from build123d import *

# Parameters (mm, degrees)
F0_R     = 11.35
F1_DEPTH = 2
F2_R     = 2.6
F3_DEPTH = 25


# Not quite as in the source:
# - a feature names something its author has since deleted; it is built from what else it names


with BuildPart() as f1:
    # F0 (on Top) → F1 (new body)
    with BuildSketch(Plane.XY):
        Circle(F0_R)
    extrude(amount=F1_DEPTH)

    # F2 (on face) → F3 (cut)
    with BuildSketch(Plane.XY.offset(2)):
        with BuildLine():
            ThreePointArc((9.1045560576, 6.7771350137), (7.7736409673, 8.2700064155), (6.2013506213, 9.506090178))
            ThreePointArc((6.2013506213, 9.506090178), (6.4038363916, 6.8127365625), (9.1045560576, 6.7771350137))
        make_face()
        with BuildLine():
            ThreePointArc((9.1045560576, 6.7771350137), (9.5987204424, 7.4520303097), (9.7736409673, 8.2700064155))
            ThreePointArc((9.7736409673, 8.2700064155), (8.4276361156, 10.1600567709), (6.2013506213, 9.506090178))
            ThreePointArc((6.2013506213, 9.506090178), (7.7736409673, 8.2700064155), (9.1045560576, 6.7771350137))
        make_face()
        with BuildLine():
            ThreePointArc((0.6174820868, 11.3331908954), (2.1395167155, 9.1019211282), (4.4962093293, 10.4214491155))
            ThreePointArc((4.4962093293, 10.4214491155), (2.5971673498, 11.0488561289), (0.6174820868, 11.3331908954))
        make_face()
        with BuildLine():
            ThreePointArc((0.6174820868, 11.3331908954), (2.5971673498, 11.0488561289), (4.4962093293, 10.4214491155))
            ThreePointArc((4.4962093293, 10.4214491155), (4.5717665445, 10.73111721), (4.5971673498, 11.0488561289))
            ThreePointArc((4.5971673498, 11.0488561289), (2.7396971257, 13.04377098), (0.6174820868, 11.3331908954))
        make_face()
        with BuildLine():
            ThreePointArc((-5.1318402741, 10.1235722648), (-3.2752151616, 10.8671737653), (-1.3168930579, 11.2733443429))
            ThreePointArc((-1.3168930579, 11.2733443429), (-3.8523455866, 12.7820942526), (-5.1318402741, 10.1235722648))
        make_face()
        with BuildLine():
            ThreePointArc((-1.2752151616, 10.8671737653), (-1.2856619194, 11.0713254155), (-1.3168930579, 11.2733443429))
            ThreePointArc((-1.3168930579, 11.2733443429), (-3.2752151616, 10.8671737653), (-5.1318402741, 10.1235722648))
            ThreePointArc((-5.1318402741, 10.1235722648), (-2.8965663963, 8.9033445689), (-1.2752151616, 10.8671737653))
        make_face()
        with BuildLine():
            ThreePointArc((-9.506090178, 6.2013506213), (-8.2700064155, 7.7736409673), (-6.7771350137, 9.1045560576))
            ThreePointArc((-6.7771350137, 9.1045560576), (-9.7272762684, 9.143445543), (-9.506090178, 6.2013506213))
        make_face()
        with BuildLine():
            ThreePointArc((-6.2700064155, 7.7736409673), (-6.4010838912, 8.4857705891), (-6.7771350137, 9.1045560576))
            ThreePointArc((-6.7771350137, 9.1045560576), (-8.2700064155, 7.7736409673), (-9.506090178, 6.2013506213))
            ThreePointArc((-9.506090178, 6.2013506213), (-7.3959833966, 5.97472914), (-6.2700064155, 7.7736409673))
        make_face()
        with BuildLine():
            ThreePointArc((-11.3331908954, 0.6174820868), (-11.0488561289, 2.5971673498), (-10.4214491155, 4.4962093293))
            ThreePointArc((-10.4214491155, 4.4962093293), (-12.9957911296, 3.0548179842), (-11.3331908954, 0.6174820868))
        make_face()
        with BuildLine():
            ThreePointArc((-9.0488561289, 2.5971673498), (-9.427928304, 3.7687444863), (-10.4214491155, 4.4962093293))
            ThreePointArc((-10.4214491155, 4.4962093293), (-11.0488561289, 2.5971673498), (-11.3331908954, 0.6174820868))
            ThreePointArc((-11.3331908954, 0.6174820868), (-9.7390220808, 1.0857657597), (-9.0488561289, 2.5971673498))
        make_face()
        with BuildLine():
            ThreePointArc((11.2733443429, 1.3168930579), (10.8671737653, 3.2752151616), (10.1235722648, 5.1318402741))
            ThreePointArc((10.1235722648, 5.1318402741), (8.952253278, 2.6980847366), (11.2733443429, 1.3168930579))
        make_face()
        with BuildLine():
            ThreePointArc((12.8671737653, 3.2752151616), (11.9880655975, 4.9315972131), (10.1235722648, 5.1318402741))
            ThreePointArc((10.1235722648, 5.1318402741), (10.8671737653, 3.2752151616), (11.2733443429, 1.3168930579))
            ThreePointArc((11.2733443429, 1.3168930579), (12.4183573707, 2.0127455887), (12.8671737653, 3.2752151616))
        make_face()
        with BuildLine():
            ThreePointArc((10.4214491155, -4.4962093293), (11.0488561289, -2.5971673498), (11.3331908954, -0.6174820868))
            ThreePointArc((11.3331908954, -0.6174820868), (9.1019211282, -2.1395167155), (10.4214491155, -4.4962093293))
        make_face()
        with BuildLine():
            ThreePointArc((13.0488561289, -2.5971673498), (12.560257719, -1.2873333018), (11.3331908954, -0.6174820868))
            ThreePointArc((11.3331908954, -0.6174820868), (11.0488561289, -2.5971673498), (10.4214491155, -4.4962093293))
            ThreePointArc((10.4214491155, -4.4962093293), (12.2204332653, -4.2180951747), (13.0488561289, -2.5971673498))
        make_face()
        with BuildLine():
            ThreePointArc((-4.4962093293, -10.4214491155), (-3.0548179842, -12.9957911296), (-0.6174820868, -11.3331908954))
            ThreePointArc((-0.6174820868, -11.3331908954), (-2.5971673498, -11.0488561289), (-4.4962093293, -10.4214491155))
        make_face()
        with BuildLine():
            ThreePointArc((-4.4962093293, -10.4214491155), (-2.5971673498, -11.0488561289), (-0.6174820868, -11.3331908954))
            ThreePointArc((-0.6174820868, -11.3331908954), (-0.6022524988, -11.1913859047), (-0.5971673498, -11.0488561289))
            ThreePointArc((-0.5971673498, -11.0488561289), (-2.2794284309, -9.0742569343), (-4.4962093293, -10.4214491155))
        make_face()
        with BuildLine():
            ThreePointArc((-10.1235722648, -5.1318402741), (-10.8671737653, -3.2752151616), (-11.2733443429, -1.3168930579))
            ThreePointArc((-11.2733443429, -1.3168930579), (-12.7820942526, -3.8523455866), (-10.1235722648, -5.1318402741))
        make_face()
        with BuildLine():
            ThreePointArc((-8.8671737653, -3.2752151616), (-9.6047041924, -1.7240315562), (-11.2733443429, -1.3168930579))
            ThreePointArc((-11.2733443429, -1.3168930579), (-10.8671737653, -3.2752151616), (-10.1235722648, -5.1318402741))
            ThreePointArc((-10.1235722648, -5.1318402741), (-9.2107917138, -4.3961069938), (-8.8671737653, -3.2752151616))
        make_face()
        with BuildLine():
            ThreePointArc((-6.2013506213, -9.506090178), (-7.7736409673, -8.2700064155), (-9.1045560576, -6.7771350137))
            ThreePointArc((-9.1045560576, -6.7771350137), (-9.143445543, -9.7272762684), (-6.2013506213, -9.506090178))
        make_face()
        with BuildLine():
            ThreePointArc((-5.7736409673, -8.2700064155), (-6.9556648615, -6.4449269404), (-9.1045560576, -6.7771350137))
            ThreePointArc((-9.1045560576, -6.7771350137), (-7.7736409673, -8.2700064155), (-6.2013506213, -9.506090178))
            ThreePointArc((-6.2013506213, -9.506090178), (-5.8835906119, -8.9240015638), (-5.7736409673, -8.2700064155))
        make_face()
        with BuildLine():
            ThreePointArc((6.7771350137, -9.1045560576), (8.2700064155, -7.7736409673), (9.506090178, -6.2013506213))
            ThreePointArc((9.506090178, -6.2013506213), (6.8127365625, -6.4038363916), (6.7771350137, -9.1045560576))
        make_face()
        with BuildLine():
            ThreePointArc((10.2700064155, -7.7736409673), (10.0689182428, -6.8996179484), (9.506090178, -6.2013506213))
            ThreePointArc((9.506090178, -6.2013506213), (8.2700064155, -7.7736409673), (6.7771350137, -9.1045560576))
            ThreePointArc((6.7771350137, -9.1045560576), (8.9821360372, -9.6425634916), (10.2700064155, -7.7736409673))
        make_face()
        with BuildLine():
            ThreePointArc((1.3168930579, -11.2733443429), (3.2752151616, -10.8671737653), (5.1318402741, -10.1235722648))
            ThreePointArc((5.1318402741, -10.1235722648), (2.6980847366, -8.952253278), (1.3168930579, -11.2733443429))
        make_face()
        with BuildLine():
            ThreePointArc((5.2752151616, -10.8671737653), (5.239044358, -10.488525), (5.1318402741, -10.1235722648))
            ThreePointArc((5.1318402741, -10.1235722648), (3.2752151616, -10.8671737653), (1.3168930579, -11.2733443429))
            ThreePointArc((1.3168930579, -11.2733443429), (3.4793668118, -12.8567270075), (5.2752151616, -10.8671737653))
        make_face()
        Circle(F2_R)
    extrude(amount=-F3_DEPTH, mode=Mode.SUBTRACT)


solid = f1.part
Check sheet for the modelled part. Datum: model origin and axes. Units: mm. Give positions to 0.01 mm unless a question says otherwise; leave off trailing zeros. Order: outer loops, then holes, each group sorted by start corner. A loop starts at its lowest first (then second) coordinate and runs counter-clockwise, first axis right, second up. Notation, with made-up numbers: M 50,20.25 L 91,20.25 A19 ccw 91,32.25 Z; hole C 2.5,47.5 d10. An arc over 180 degrees is marked long. Answer as CSV lines item,"result". Start each with the question number.
Item 1: Thickness scan on line 1 (Y direction, x = 10, z = 1.5); line 2 (Y direction, x = 0, z = 0.7); line 3 (X direction, y = -1.75, z = 0.95). Record the ranges inside material, lowest first. Write a range as [from, to].
Item 2: Cross-section at A-A on y = 0. Enter the section's corners in (x, z), plus the area to 3 significant figures.
Item 3: Cross-section at D-D on y = 3.75. Enter the section's corners in (x, z), plus the area to 3 significant figures.
Item 4: Gauge pin test, flat end, axial feed: P1, Ø6, axis at x = -9, y = -3.5, coming from the -Z side. Record the tip position at first contact, or that the pin passes through.
Item 5: Mould release check, pull along Y, two halves, no side actions. Record for faces 1 (the face through (0, 3, 2)), 2 (the face through (5.38, 9.994, 0.986)), 3 (the face through (6.374, 6.841, 1.014)), 4 (the face through (0.337, -11.345, 0.986)): +Y half, -Y half, draft (parallel to the pull), parting line (faces both ways), or undercut.
Item 6: Cross-section at C-C on z = 0.3. Enter the section's corners in (x, y), plus the area to 3 significant figures.
Established:
1,line 1,"y = [-5.37, -4.3], [-0.89, 1.47], [5.08, 5.37]"
1,line 2,"y = [-11.35, -2.6], [2.6, 11.35]"
1,line 3,"x = [-9.57, -1.92], [1.92, 9.24]"
2,outline,"M -11.35,0 L -2.6,0 L -2.6,2 L -11.35,2 Z; M 2.6,0 L 11.35,0 L 11.35,2 L 2.6,2 Z"
2,area,"35.0 mm^2"
3,outline,"M -9.41,0 L 8.92,0 L 8.92,2 L -9.41,2 Z"
3,area,"36.7 mm^2"
4,P1,"stops at z = 0"
5,face 1,"draft"
5,face 2,"+Y half"
5,face 3,"undercut"
5,face 4,"-Y half"
6,outline,"M -11.33,0.62 A11.35 ccw -11.27,-1.32 A2 cw -10.12,-5.13 A11.35 ccw -9.1,-6.78 A2 cw -6.2,-9.51 A11.35 ccw -4.5,-10.42 A2 cw -0.62,-11.33 A11.35 ccw 1.32,-11.27 A2 cw 5.13,-10.12 A11.35 ccw 6.78,-9.1 A2 cw 9.51,-6.2 A11.35 ccw 10.42,-4.5 A2 cw 11.33,-0.62 A11.35 ccw 11.27,1.32 A2 cw 10.12,5.13 A11.35 ccw 9.1,6.78 A2 cw 6.2,9.51 A11.35 ccw 4.5,10.42 A2 cw 0.62,11.33 A11.35 ccw -1.32,11.27 A2 cw -5.13,10.12 A11.35 ccw -6.78,9.1 A2 cw -9.51,6.2 A11.35 ccw -10.42,4.5 A2 cw Z; hole C 0,0 d5.2"
6,area,"311 mm^2"
